from build123d import *

# Parameters (mm, degrees)
EXTRUDE1_DEPTH          = 1.25
CUT_EXTRUDE3_DEPTH      = 2.25
LPATTERN4_COUNT         = 2
LPATTERN4_PITCH         = 2.54
SKETCH2_W               = 1.752893218
SKETCH2_H               = 0.33
CUT_EXTRUDE1_DEPTH      = 2.27
CUT_EXTRUDE1_DEPTH_BACK = 4.81
EXTRUDE_THIN1_DEPTH     = 0.32
LPATTERN5_COUNT         = 2
LPATTERN5_PITCH         = 2.54
CHAMFER2_SIZE           = 0.6
CHAMFER2_SIZE2          = 0.105796188
CHAMFER2_PART_2_SIZE    = 0.6
CHAMFER2_PART_2_SIZE2   = 0.105796188
CHAMFER2_PART_3_SIZE    = 0.6
CHAMFER2_PART_3_SIZE2   = 0.105796188
CHAMFER2_PART_4_SIZE    = 0.6
CHAMFER2_PART_4_SIZE2   = 0.105796188
CHAMFER2_PART_5_SIZE    = 0.6
CHAMFER2_PART_5_SIZE2   = 0.105796188
CHAMFER2_PART_6_SIZE    = 0.6
CHAMFER2_PART_6_SIZE2   = 0.105796188
CHAMFER2_PART_7_SIZE    = 0.6
CHAMFER2_PART_7_SIZE2   = 0.105796188
CHAMFER2_PART_8_SIZE    = 0.6
CHAMFER2_PART_8_SIZE2   = 0.105796188
CHAMFER2_PART_9_SIZE    = 0.6
CHAMFER2_PART_9_SIZE2   = 0.105796188
CHAMFER2_PART_10_SIZE   = 0.6
CHAMFER2_PART_10_SIZE2  = 0.105796188
CHAMFER2_PART_11_SIZE   = 0.6
CHAMFER2_PART_11_SIZE2  = 0.105796188
CHAMFER2_PART_12_SIZE   = 0.6
CHAMFER2_PART_12_SIZE2  = 0.105796188
CHAMFER2_PART_13_SIZE   = 0.6
CHAMFER2_PART_13_SIZE2  = 0.105796188
CHAMFER2_PART_14_SIZE   = 0.6
CHAMFER2_PART_14_SIZE2  = 0.105796188
CHAMFER2_PART_15_SIZE   = 0.6
CHAMFER2_PART_15_SIZE2  = 0.105796188
CHAMFER2_PART_16_SIZE   = 0.6
CHAMFER2_PART_16_SIZE2  = 0.105796188
FILLET1_R               = 0.5
FILLET2_R               = 1.14


with BuildPart() as part:
    # Sketch1 → Extrude1 (new body, symmetric)
    with BuildSketch(Plane.XY):
        Polygon((-1.27, 0.896446609), (-0.916446609, 1.25), (0.916446609, 1.25), (1.27, 0.896446609), (1.27, -0.896446609), (0.916446609, -1.25), (-0.916446609, -1.25), (-1.27, -0.896446609), align=None)
    extrude1 = extrude(amount=EXTRUDE1_DEPTH, both=True)

    # Sketch4 → Cut-Extrude3 (cut, symmetric)
    with BuildSketch(Plane(origin=(0, 0, 0), x_dir=(1, 0, 0), z_dir=(0, 1, 0))):
        Polygon((-1.27, -1.15), (-1.17, -1.25), (-1.27, -1.25), align=None)
        Polygon((1.17, -1.25), (1.27, -1.15), (1.27, -1.25), align=None)
    cut_extrude3 = extrude(amount=CUT_EXTRUDE3_DEPTH, both=True, mode=Mode.SUBTRACT)

    # LPattern4: Extrude1, Cut-Extrude3 ×2
    with Locations(*[(-i * LPATTERN4_PITCH, 0, 0) for i in range(1, LPATTERN4_COUNT)]):
        add(extrude1)
        add(cut_extrude3, mode=Mode.SUBTRACT)

    # Sketch2 → Cut-Extrude1 (cut, two sides)
    with BuildSketch(Plane(origin=(0, 0, 0), x_dir=(0, -1, 0), z_dir=(1, 0, 0))) as cut_extrude1_sk:
        with Locations((0, 1.085)):
            Rectangle(SKETCH2_W, SKETCH2_H)
    extrude(amount=CUT_EXTRUDE1_DEPTH, mode=Mode.SUBTRACT)
    extrude(cut_extrude1_sk.sketch, amount=-CUT_EXTRUDE1_DEPTH_BACK, mode=Mode.SUBTRACT)

    # Sketch3 → Extrude-Thin1 (add, symmetric)
    with BuildSketch(Plane(origin=(0, 0, 0), x_dir=(0, 0, -1), z_dir=(1, 0, 0))):
        Polygon((-7.25, -0.32), (2.43, -0.32), (2.43, -3.25), (3.07, -3.25), (3.07, 0.32), (-7.25, 0.32), align=None)
    extrude_thin1 = extrude(amount=EXTRUDE_THIN1_DEPTH, both=True)

    # LPattern5: Extrude-Thin1 ×2
    with Locations(*[(-i * LPATTERN5_PITCH, 0, 0) for i in range(1, LPATTERN5_COUNT)]):
        add(extrude_thin1)

    # Chamfer2
    chamfer2_edges = [part.edges().sort_by_distance(p)[0] for p in [
        (0, -0.32, 7.25),
    ]]
    chamfer2_side = [part.faces().sort_by_distance(p)[0] for p in [
        (0, -0.32, 4.25),
    ]]
    chamfer(chamfer2_edges, length=CHAMFER2_SIZE, length2=CHAMFER2_SIZE2, reference=chamfer2_side[0])

    # Chamfer2 part 2
    chamfer2_part_2_edges = [part.edges().sort_by_distance(p)[0] for p in [
        (-0.32, 0, 7.25),
    ]]
    chamfer2_part_2_side = [part.faces().sort_by_distance(p)[0] for p in [
        (-0.32, 0, 4.25),
    ]]
    chamfer(chamfer2_part_2_edges, length=CHAMFER2_PART_2_SIZE, length2=CHAMFER2_PART_2_SIZE2, reference=chamfer2_part_2_side[0])

    # Chamfer2 part 3
    chamfer2_part_3_edges = [part.edges().sort_by_distance(p)[0] for p in [
        (-0.32, -3.25, -2.75),
    ]]
    chamfer2_part_3_side = [part.faces().sort_by_distance(p)[0] for p in [
        (-0.32, -1.029537402, -2.430462598),
    ]]
    chamfer(chamfer2_part_3_edges, length=CHAMFER2_PART_3_SIZE, length2=CHAMFER2_PART_3_SIZE2, reference=chamfer2_part_3_side[0])

    # Chamfer2 part 4
    chamfer2_part_4_edges = [part.edges().sort_by_distance(p)[0] for p in [
        (0, -3.25, -2.43),
    ]]
    chamfer2_part_4_side = [part.faces().sort_by_distance(p)[0] for p in [
        (0, -1.785, -2.43),
    ]]
    chamfer(chamfer2_part_4_edges, length=CHAMFER2_PART_4_SIZE, length2=CHAMFER2_PART_4_SIZE2, reference=chamfer2_part_4_side[0])

    # Chamfer2 part 5
    chamfer2_part_5_edges = [part.edges().sort_by_distance(p)[0] for p in [
        (0.32, -3.25, -2.75),
    ]]
    chamfer2_part_5_side = [part.faces().sort_by_distance(p)[0] for p in [
        (0.32, -1.029537402, -2.430462598),
    ]]
    chamfer(chamfer2_part_5_edges, length=CHAMFER2_PART_5_SIZE, length2=CHAMFER2_PART_5_SIZE2, reference=chamfer2_part_5_side[0])

    # Chamfer2 part 6
    chamfer2_part_6_edges = [part.edges().sort_by_distance(p)[0] for p in [
        (0, -3.25, -3.07),
    ]]
    chamfer2_part_6_side = [part.faces().sort_by_distance(p)[0] for p in [
        (0, -1.465, -3.07),
    ]]
    chamfer(chamfer2_part_6_edges, length=CHAMFER2_PART_6_SIZE, length2=CHAMFER2_PART_6_SIZE2, reference=chamfer2_part_6_side[0])

    # Chamfer2 part 7
    chamfer2_part_7_edges = [part.edges().sort_by_distance(p)[0] for p in [
        (0, 0.32, 7.25),
    ]]
    chamfer2_part_7_side = [part.faces().sort_by_distance(p)[0] for p in [
        (0, 0.32, 4.25),
    ]]
    chamfer(chamfer2_part_7_edges, length=CHAMFER2_PART_7_SIZE, length2=CHAMFER2_PART_7_SIZE2, reference=chamfer2_part_7_side[0])

    # Chamfer2 part 8
    chamfer2_part_8_edges = [part.edges().sort_by_distance(p)[0] for p in [
        (0.32, 0, 7.25),
    ]]
    chamfer2_part_8_side = [part.faces().sort_by_distance(p)[0] for p in [
        (0.32, 0, 4.25),
    ]]
    chamfer(chamfer2_part_8_edges, length=CHAMFER2_PART_8_SIZE, length2=CHAMFER2_PART_8_SIZE2, reference=chamfer2_part_8_side[0])

    # Chamfer2 part 9
    chamfer2_part_9_edges = [part.edges().sort_by_distance(p)[0] for p in [
        (-2.54, -0.32, 7.25),
    ]]
    chamfer2_part_9_side = [part.faces().sort_by_distance(p)[0] for p in [
        (-2.54, -0.32, 4.25),
    ]]
    chamfer(chamfer2_part_9_edges, length=CHAMFER2_PART_9_SIZE, length2=CHAMFER2_PART_9_SIZE2, reference=chamfer2_part_9_side[0])

    # Chamfer2 part 10
    chamfer2_part_10_edges = [part.edges().sort_by_distance(p)[0] for p in [
        (-2.86, 0, 7.25),
    ]]
    chamfer2_part_10_side = [part.faces().sort_by_distance(p)[0] for p in [
        (-2.86, 0, 4.25),
    ]]
    chamfer(chamfer2_part_10_edges, length=CHAMFER2_PART_10_SIZE, length2=CHAMFER2_PART_10_SIZE2, reference=chamfer2_part_10_side[0])

    # Chamfer2 part 11
    chamfer2_part_11_edges = [part.edges().sort_by_distance(p)[0] for p in [
        (-2.86, -3.25, -2.75),
    ]]
    chamfer2_part_11_side = [part.faces().sort_by_distance(p)[0] for p in [
        (-2.86, -1.029537402, -2.430462598),
    ]]
    chamfer(chamfer2_part_11_edges, length=CHAMFER2_PART_11_SIZE, length2=CHAMFER2_PART_11_SIZE2, reference=chamfer2_part_11_side[0])

    # Chamfer2 part 12
    chamfer2_part_12_edges = [part.edges().sort_by_distance(p)[0] for p in [
        (-2.54, -3.25, -2.43),
    ]]
    chamfer2_part_12_side = [part.faces().sort_by_distance(p)[0] for p in [
        (-2.54, -1.785, -2.43),
    ]]
    chamfer(chamfer2_part_12_edges, length=CHAMFER2_PART_12_SIZE, length2=CHAMFER2_PART_12_SIZE2, reference=chamfer2_part_12_side[0])

    # Chamfer2 part 13
    chamfer2_part_13_edges = [part.edges().sort_by_distance(p)[0] for p in [
        (-2.22, -3.25, -2.75),
    ]]
    chamfer2_part_13_side = [part.faces().sort_by_distance(p)[0] for p in [
        (-2.22, -1.029537402, -2.430462598),
    ]]
    chamfer(chamfer2_part_13_edges, length=CHAMFER2_PART_13_SIZE, length2=CHAMFER2_PART_13_SIZE2, reference=chamfer2_part_13_side[0])

    # Chamfer2 part 14
    chamfer2_part_14_edges = [part.edges().sort_by_distance(p)[0] for p in [
        (-2.54, -3.25, -3.07),
    ]]
    chamfer2_part_14_side = [part.faces().sort_by_distance(p)[0] for p in [
        (-2.54, -1.465, -3.07),
    ]]
    chamfer(chamfer2_part_14_edges, length=CHAMFER2_PART_14_SIZE, length2=CHAMFER2_PART_14_SIZE2, reference=chamfer2_part_14_side[0])

    # Chamfer2 part 15
    chamfer2_part_15_edges = [part.edges().sort_by_distance(p)[0] for p in [
        (-2.54, 0.32, 7.25),
    ]]
    chamfer2_part_15_side = [part.faces().sort_by_distance(p)[0] for p in [
        (-2.54, 0.32, 4.25),
    ]]
    chamfer(chamfer2_part_15_edges, length=CHAMFER2_PART_15_SIZE, length2=CHAMFER2_PART_15_SIZE2, reference=chamfer2_part_15_side[0])

    # Chamfer2 part 16
    chamfer2_part_16_edges = [part.edges().sort_by_distance(p)[0] for p in [
        (-2.22, 0, 7.25),
    ]]
    chamfer2_part_16_side = [part.faces().sort_by_distance(p)[0] for p in [
        (-2.22, 0, 4.25),
    ]]
    chamfer(chamfer2_part_16_edges, length=CHAMFER2_PART_16_SIZE, length2=CHAMFER2_PART_16_SIZE2, reference=chamfer2_part_16_side[0])

    # Fillet1
    fillet1_edges = [part.edges().sort_by_distance(p)[0] for p in [
        (0, -0.32, -2.43),
        (-2.54, -0.32, -2.43),
    ]]
    fillet(fillet1_edges, radius=FILLET1_R)

    # Fillet2
    fillet2_edges = [part.edges().sort_by_distance(p)[0] for p in [
        (0, 0.32, -3.07),
        (-2.54, 0.32, -3.07),
    ]]
    fillet(fillet2_edges, radius=FILLET2_R)


solid = part.part
Build history of the part. All positions in model axes, mm. A direction names the side the tool comes from. Coordinates: 2 decimals unless noted, no trailing zeros. Write each loop counter-clockwise with the first axis right and the second up, starting at its lowest first coordinate (ties: lowest second). Pieces come first, ordered by that corner, then holes.
(1) 3-axis set-ups, long thin cutter, end or side, ignore diameter. For faces 1 (the flat face through (0, 1.25, 0)), 2 (the flat face through (-3.04, 0.02, 1.25)), 3 (the flat face through (0, -1.25, 0)): which of +Z, -Z, +X, -X, +Y, -Y reach the whole face in a straight line?
(2) Cut at A-A on z = 6.25. List the corners of the cut face in (x, y).
(3) Cut at C-C on y = -0.7. List the corners of the cut face in (x, z).
(4) Cut at D-D on z = 0. List the corners of the cut face in (x, y).
(5) Cut at B-B on x = -2.5. List the corners of the cut face in (y, z), and give its area (3 significant figures).
(6) Pin check, flat tips, straight feed: pin 1 Ø1.5 at (y, z) = (0, -2) entering from +X; pin 2 Ø0.5 at (x, z) = (-2.5, -1) entering from -Y; pin 3 Ø0.6 at (y, z) = (-1.5, -2.5) entering from -X. Stop position of each tip, or through.
(7) Mould opens along X. For faces 4 (the flat face through (-2.86, -0.8, -2.7)), 5 (the cylindrical face through (-2.54, -0.02, -2.74)), 6 (the flat face through (-1, 0, -0.92)) say: pulls with the +X half, pulls with the -X half, needs draft (parallel to the pull), parting line crosses it, or undercut.
(8) Drill centre lines: line 1 (Y direction, x = -2.5, z = -1); line 2 (Z direction, x = -2.6, y = -1.45); line 3 (Y direction, x = -0.15, z = 5.25). Where is each one in solid material? Low to high.
Working result:
1. face 1: +Z, -Z, +X, -X, +Y
1. face 2: +Z
1. face 3: +Z, +X, -X, -Y
2. outline: (-2.86, -0.32) - (-2.22, -0.32) - (-2.22, 0.32) - (-2.86, 0.32) - close; (-0.32, -0.32) - (0.32, -0.32) - (0.32, 0.32) - (-0.32, 0.32) - close
3. outline: (-3.81, -0.92) - (1.27, -0.92) - (1.27, 1.15) - (1.17, 1.25) - (-1.17, 1.25) - (-1.27, 1.15) - (-1.37, 1.25) - (-3.71, 1.25) - (-3.81, 1.15) - close; (-2.86, -3.06) - (-2.22, -3.06) - (-2.22, -2.42) - (-2.86, -2.42) - close; (-0.32, -3.06) - (0.32, -3.06) - (0.32, -2.42) - (-0.32, -2.42) - close
4. outline: (-3.81, -0.9) - (-3.46, -1.25) - (-1.62, -1.25) - (-1.27, -0.9) - (-0.92, -1.25) - (0.92, -1.25) - (1.27, -0.9) - (1.27, 0.9) - (0.92, 1.25) - (-0.92, 1.25) - (-1.27, 0.9) - (-1.62, 1.25) - (-3.46, 1.25) - (-3.81, 0.9) - close
5. outline: (-3.25, -2.96) - (-2.65, -3.07) - (-0.82, -3.07) arc R1.14 ccw to (0.32, -1.93) - (0.32, -0.92) - (0.88, -0.92) - (0.88, -1.25) - (1.25, -1.25) - (1.25, 1.25) - (0.32, 1.25) - (0.32, 6.65) - (0.21, 7.25) - (-0.21, 7.25) - (-0.32, 6.65) - (-0.32, 1.25) - (-1.25, 1.25) - (-1.25, -1.25) - (-0.88, -1.25) - (-0.88, -0.92) - (-0.32, -0.92) - (-0.32, -1.93) arc R0.5 cw to (-0.82, -2.43) - (-2.65, -2.43) - (-3.25, -2.54) - close
5. area: 12.4 mm2
6. pin 1: stops at x = 0.32
6. pin 2: stops at y = -1.25
6. pin 3: stops at x = -2.86
7. face 4: pulls with the -X half
7. face 5: needs draft
7. face 6: undercut
8. line 1: y = -1.25 to -0.88, -0.32 to 0.32, 0.88 to 1.25
8. line 2: z = -3.07 to -2.43
8. line 3: y = -0.32 to 0.32
